```python
from build123d import *

# Parameters (mm, degrees)
F0_R          = 25.4
F1_DEPTH      = 6.35
F2_DEPTH      = 31.75
F2_DEPTH_BACK = 3.175
F3_DEPTH      = 12.7


with BuildPart() as f1:
    # F0 (on Front) → F1 (new body)
    with BuildSketch(Plane.XZ):
        with BuildLine():
            ThreePointArc((50.7756672677, -1.5721366092), (45.94665551, 2.8907185428), (50.1782450005, 7.9236184075))
            ThreePointArc((50.1782450005, 7.9236184075), (49.900192337, 9.518970781), (49.5714307865, 11.1046499169))
            ThreePointArc((49.5714307865, 11.1046499169), (43.7842643689, 14.2263698785), (46.6312793948, 20.153505452))
            ThreePointArc((46.6312793948, 20.153505452), (45.9652142653, 21.6295880115), (45.2524389981, 23.0836904486))
            ThreePointArc((45.2524389981, 23.0836904486), (38.8707468703, 24.6681260738), (40.1542990068, 31.1170736296))
            ThreePointArc((40.1542990068, 31.1170736296), (39.142072733, 32.3811386792), (38.0900700405, 33.6122978136))
            ThreePointArc((38.0900700405, 33.6122978136), (31.5148373892, 33.5598931849), (31.1542763351, 40.1254416304))
            ThreePointArc((31.1542763351, 40.1254416304), (29.8594908165, 41.0980633142), (28.5343618968, 42.0289208896))
            ThreePointArc((28.5343618968, 42.0289208896), (22.1787347715, 40.3429687825), (20.1967159038, 46.6125805626))
            ThreePointArc((20.1967159038, 46.6125805626), (18.7007272764, 47.2326454831), (17.1857348531, 47.8047122945))
            ThreePointArc((17.1857348531, 47.8047122945), (11.4490606804, 44.5911472805), (7.970121534, 50.1708796289))
            ThreePointArc((7.970121534, 50.1708796289), (6.3669282651, 50.3994268268), (4.7572648839, 50.5767578125))
            ThreePointArc((4.7572648839, 50.5767578125), (0, 46.0375), (-4.7572648839, 50.5767578125))
            ThreePointArc((-4.7572648839, 50.5767578125), (-6.3669282651, 50.3994268268), (-7.970121534, 50.1708796289))
            ThreePointArc((-7.970121534, 50.1708796289), (-7.8958049616, 49.6899886809), (-7.870946268, 49.2040245853))
            ThreePointArc((-7.870946268, 49.2040245853), (-11.9259394259, 44.4943706364), (-17.1857348531, 47.8047122945))
            ThreePointArc((-17.1857348531, 47.8047122945), (-18.7007272764, 47.2326454831), (-20.1967159038, 46.6125805626))
            ThreePointArc((-20.1967159038, 46.6125805626), (-19.8337105062, 45.5922953741), (-19.7105866444, 44.5163793462))
            ThreePointArc((-19.7105866444, 44.5163793462), (-23.1808825467, 39.9325365457), (-28.5343618968, 42.0289208896))
            ThreePointArc((-28.5343618968, 42.0289208896), (-29.8594908165, 41.0980633142), (-31.1542763351, 40.1254416304))
            ThreePointArc((-31.1542763351, 40.1254416304), (-30.3070477444, 38.6805063948), (-30.0124929812, 37.031606273))
            ThreePointArc((-30.0124929812, 37.031606273), (-32.9184704584, 32.6458645601), (-38.0900700405, 33.6122978136))
            ThreePointArc((-38.0900700405, 33.6122978136), (-39.142072733, 32.3811386792), (-40.1542990068, 31.1170736296))
            ThreePointArc((-40.1542990068, 31.1170736296), (-38.6658064456, 29.4158812606), (-38.1293586155, 27.2200011849))
            ThreePointArc((-38.1293586155, 27.2200011849), (-40.5002961369, 23.1015263263), (-45.2524389981, 23.0836904486))
            ThreePointArc((-45.2524389981, 23.0836904486), (-45.9652142653, 21.6295880115), (-46.6312793948, 20.153505452))
            ThreePointArc((-46.6312793948, 20.153505452), (-44.3961592919, 18.4062930033), (-43.5511710278, 15.6980633142))
            ThreePointArc((-43.5511710278, 15.6980633142), (-45.4247849623, 11.9118061187), (-49.5714307865, 11.1046499169))
            ThreePointArc((-49.5714307865, 11.1046499169), (-49.900192337, 9.518970781), (-50.1782450005, 7.9236184075))
            ThreePointArc((-50.1782450005, 7.9236184075), (-47.1525680025, 6.3676272946), (-45.9372578042, 3.1897583921))
            ThreePointArc((-45.9372578042, 3.1897583921), (-47.3591076107, -0.2045696025), (-50.7756672677, -1.5721366092))
            ThreePointArc((-50.7756672677, -1.5721366092), (-50.6997578042, -3.1897583921), (-50.5723269302, -4.8041387226))
            ThreePointArc((-50.5723269302, -4.8041387226), (-46.7792657719, -5.9215795561), (-45.137692337, -9.518970781))
            ThreePointArc((-45.137692337, -9.518970781), (-46.1604620648, -12.4678389946), (-48.7894818346, -14.1501400102))
            ThreePointArc((-48.7894818346, -14.1501400102), (-48.3136710278, -15.6980633142), (-47.7887635668, -17.2300341484))
            ThreePointArc((-47.7887635668, -17.2300341484), (-43.3197698129, -17.6694074728), (-41.2027142653, -21.6295880115))
            ThreePointArc((-41.2027142653, -21.6295880115), (-41.8853816947, -24.0864910308), (-43.7376738227, -25.8390380738))
            ThreePointArc((-43.7376738227, -25.8390380738), (-42.8918586155, -27.2200011849), (-42.0024564338, -28.5733031609))
            ThreePointArc((-42.0024564338, -28.5733031609), (-37.0138306327, -28.1206232395), (-34.379572733, -32.3811386792))
            ThreePointArc((-34.379572733, -32.3811386792), (-34.7864792609, -34.3073296759), (-35.9376669086, -35.9043743458))
            ThreePointArc((-35.9376669086, -35.9043743458), (-34.7749929812, -37.031606273), (-33.5769804888, -38.1212064507))
            ThreePointArc((-33.5769804888, -38.1212064507), (-28.2820147175, -36.604403847), (-25.0969908165, -41.0980633142))
            ThreePointArc((-25.0969908165, -41.0980633142), (-25.2968267537, -42.4631651056), (-25.8795642131, -43.7137067307))
            ThreePointArc((-25.8795642131, -43.7137067307), (-24.4730866444, -44.5163793462), (-23.0417393722, -45.2738141391))
            ThreePointArc((-23.0417393722, -45.2738141391), (-17.6988949192, -42.5767096827), (-13.9382272764, -47.2326454831))
            ThreePointArc((-13.9382272764, -47.2326454831), (-14.0029485609, -48.0151295985), (-14.1953533198, -48.7763461539))
            ThreePointArc((-14.1953533198, -48.7763461539), (-12.633446268, -49.2040245853), (-11.0587010292, -49.5817015798))
            ThreePointArc((-11.0587010292, -49.5817015798), (-5.9565391444, -45.6546415819), (-1.6044282651, -50.3994268268))
            ThreePointArc((-1.6044282651, -50.3994268268), (-1.6081216736, -50.5869530242), (-1.6191961705, -50.7741883614))
            ThreePointArc((-1.6191961705, -50.7741883614), (0, -50.8), (1.6191961705, -50.7741883614))
            ThreePointArc((1.6191961705, -50.7741883614), (5.7700287402, -45.6744805618), (11.0587010292, -49.5817015798))
            ThreePointArc((11.0587010292, -49.5817015798), (12.633446268, -49.2040245853), (14.1953533198, -48.7763461539))
            ThreePointArc((14.1953533198, -48.7763461539), (16.9475340942, -42.8045849691), (23.0417393722, -45.2738141391))
            ThreePointArc((23.0417393722, -45.2738141391), (24.4730866444, -44.5163793462), (25.8795642131, -43.7137067307))
            ThreePointArc((25.8795642131, -43.7137067307), (27.0601635524, -37.2451198785), (33.5769804888, -38.1212064507))
            ThreePointArc((33.5769804888, -38.1212064507), (34.7749929812, -37.031606273), (35.9376669086, -35.9043743458))
            ThreePointArc((35.9376669086, -35.9043743458), (35.4725034143, -29.3454069281), (42.0024564338, -28.5733031609))
            ThreePointArc((42.0024564338, -28.5733031609), (42.8918586155, -27.2200011849), (43.7376738227, -25.8390380738))
            ThreePointArc((43.7376738227, -25.8390380738), (41.6559754279, -19.6018141354), (47.7887635668, -17.2300341484))
            ThreePointArc((47.7887635668, -17.2300341484), (48.3136710278, -15.6980633142), (48.7894818346, -14.1501400102))
            ThreePointArc((48.7894818346, -14.1501400102), (45.2220493054, -8.6265672702), (50.5723269302, -4.8041387226))
            ThreePointArc((50.5723269302, -4.8041387226), (50.6997578042, -3.1897583921), (50.7756672677, -1.5721366092))
        make_face()
        Circle(F0_R, mode=Mode.SUBTRACT)
    extrude(amount=F1_DEPTH)

    # F0 (on Front) → F2 (join, two sides)
    with BuildSketch(Plane.XZ) as f2_sk:
        Circle(F0_R)
    extrude(amount=F2_DEPTH)
    extrude(f2_sk.sketch, amount=-F2_DEPTH_BACK)

    # F3 (add): a face of the model
    f3_faces = [f1.faces().sort_by_distance(p)[0] for p in [
        (0, 3.175, 0),
    ]]
    extrude(f3_faces, amount=F3_DEPTH)


solid = f1.part
```
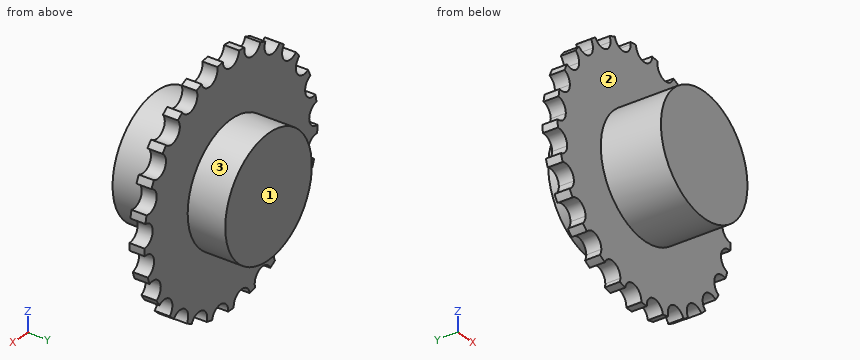
Work out the finished part from the listing and answer in its coordinate system (mm). Face numbers are marked on the shaded views. A direction names the side the tool comes from. Round coordinates to 2 decimals unless told otherwise and drop trailing zeros. Write each loop counter-clockwise with the first axis right and the second up, starting at its lowest first coordinate (ties: lowest second). Pieces come first, ordered by that corner, then holes. Notation, with made-up numbers: (13.25, 68) - (23.25, 68) arc R16 cw to (23.25, 97) - close; hole circle Ø11 at (58, 37.5). An arc over 180 degrees is marked (long way). Return JSON: item names as keys, results as strings. Group by question number.
Q1. The part is cut by section D-D on z = -30. Write down the section's boundary in (x, y).
Q2. For the marked faces 1, 2 and 3, determine the directions among +Z, -Z, +X, -X, +Y, -Y from which every point of the face is accessible in a straight line to the end or side of a thin tool.
Q3. Each of these flat-tipped pins is pushed along its axis until it touches: pin 1 Ø1 at (y, z) = (-22.5, 14) entering from -X; pin 2 Ø1.5 at (y, z) = (-1.5, 15.5) entering from -X; pin 3 Ø10 at (y, z) = (10.5, -10.5) entering from -X. Where does it stop, or does it pass through?
Q4. Find the intervals of material crossed by L1, parallel to Y at x = -30.5, z = 40.5; L2, parallel to X at y = -1, z = -32; L3, parallel to X at y = -3, z = -45, in increasing order.
Q5. The part is cut by section B-B on z = 0. Write down the section's boundary in (x, y) (3 decimals), then the cut area to 3 significant figures.
Q6. The part is cut by section C-C on y = -17. Write down the section's boundary in (x, z).
Solved:
{
 "1": {"outline": "(-35.02, -6.35) - (35.02, -6.35) - (35.02, 0) - (-35.02, 0) - close"},
 "2": {"face 1": "+Z, -Z, +X, -X, +Y", "face 2": "-Y", "face 3": "+Y"},
 "3": {"pin 1": "x = -21.52", "pin 2": "x = -43.65", "pin 3": "x = -24.8"},
 "4": {"L1": "-6.35 to 0", "L2": "-34.39 to 34.39", "L3": "-23.57 to -22.91, -14.49 to 14.49, 22.91 to 23.57"},
 "5": {"outline": "(-47.163, -6.35) - (-25.4, -6.35) - (-25.4, -31.75) - (25.4, -31.75) - (25.4, -6.35) - (47.163, -6.35) - (47.163, 0) - (25.4, 0) - (25.4, 15.875) - (-25.4, 15.875) - (-25.4, 0) - (-47.163, 0) - close", "area": "2,700 mm²"},
 "6": {"outline": "circle Ø50.8 at (0, 0)"}
}
